The drawing under review shows one solid part. Ordinate dimensions are in mm from its lowest x, y, z. A direction names the side the tool comes from. Give positions to 0.01 mm unless a question says otherwise; leave off trailing zeros. Write each loop counter-clockwise with the first axis right and the second up, starting at its lowest first coordinate (ties: lowest second). Pieces come first, ordered by that corner, then holes. Notation, with made-up numbers: (-39.5, 16) -> (-31.5, 16) arc R35 ccw to (-31.5, 53) -> close; hole circle Ø4 at (-17.75, 17). An arc over 180 degrees is marked (long way). Answer as a JSON object with one key per item and string values.
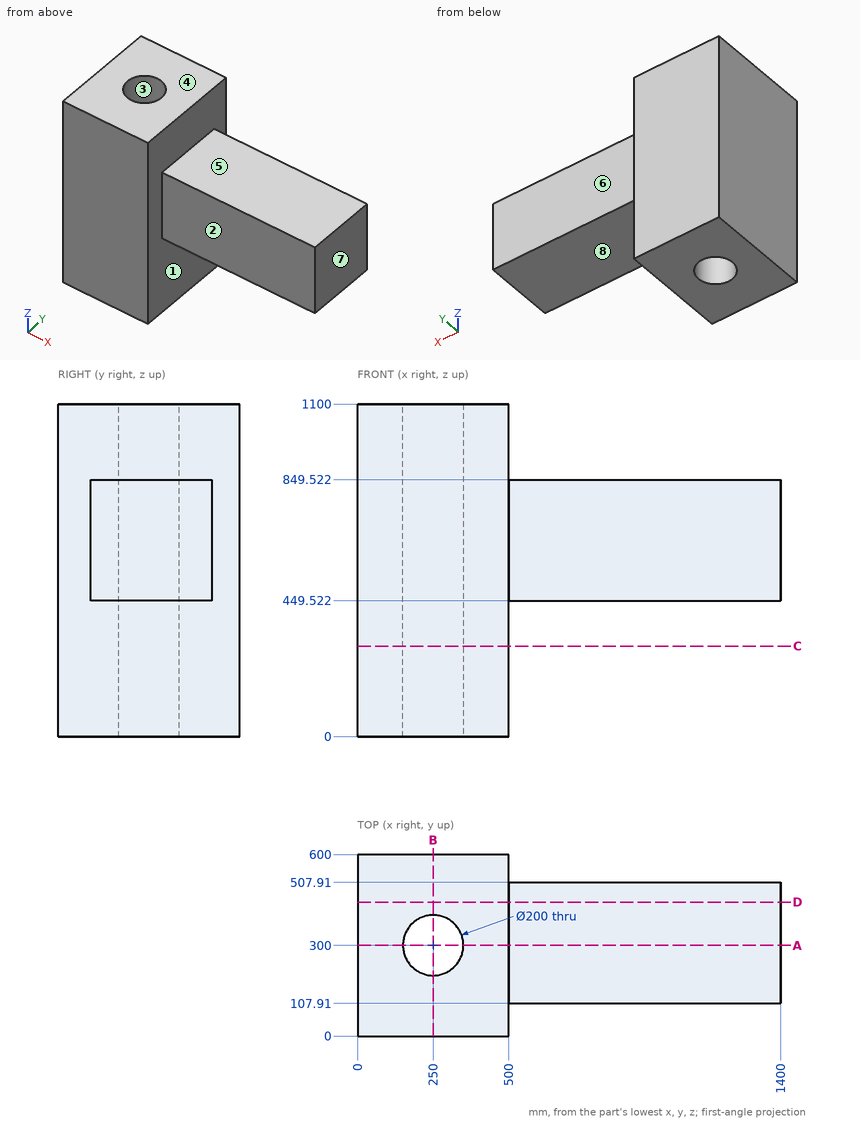
(1) For the marked faces 4, 5, 6, 7 and 8, list the 3-axis set-ups (+Z, -Z, +X, -X, +Y, -Y) from which the entire face can be reached by the end or side of a thin tool; tool diameter is ignored.
Here are the results:
{"face 4": "+Z, +X, -X, +Y, -Y", "face 5": "+Z, +X, +Y, -Y", "face 6": "+Z, -Z, +X, +Y", "face 7": "+Z, -Z, +X, +Y, -Y", "face 8": "-Z, +X, +Y, -Y"}
(2) For line 1 along Y through (x, z) = (250, 843); line 2 along X through (y, z) = (302.5, 296); line 3 along Z through (x, y) = (937, 423.5), list the stretches that pass through material, from the lowest coordinate up.
Here are the results:
{"line 1": "y = 0 to 200, 400 to 600", "line 2": "x = 0 to 150.03, 349.97 to 500", "line 3": "z = 449.52 to 849.52"}
(3) We need section D-D, the plane y = 443. State the section outline as (x, z) points.
Here are the results:
{"outline": "(0, 0) -> (500, 0) -> (500, 449.52) -> (1400, 449.52) -> (1400, 849.52) -> (500, 849.52) -> (500, 1100) -> (0, 1100) -> close"}
(4) The part is to be moulded in two halves that separate along Y. For the marked faces 1, 2 and 3, say which applies: +Y half, -Y half, draft (parallel to the pull), parting line (faces both ways), or undercut.
Here are the results:
{"face 1": "draft", "face 2": "-Y half", "face 3": "undercut"}
(5) We need section A-A, the plane y = 300. State the section outline as (x, z) points.
Here are the results:
{"outline": "(0, 0) -> (150, 0) -> (150, 1100) -> (0, 1100) -> close; (350, 0) -> (500, 0) -> (500, 449.52) -> (1400, 449.52) -> (1400, 849.52) -> (500, 849.52) -> (500, 1100) -> (350, 1100) -> close"}
(6) We need section C-C, the plane z = 299.5. State the section outline as (x, y) points.
Here are the results:
{"outline": "(0, 0) -> (500, 0) -> (500, 600) -> (0, 600) -> close; hole circle Ø200 at (250, 300)"}
(7) Clearance check with flat-ended pins moving along their axes: pin 1 (6 mm diameter, centred on x = 846, z = 743.5, fed in from +Y); pin 2 (6 mm diameter, centred on x = 696.5, y = 209.5, fed in from -Z); pin 3 (4 mm diameter, centred on x = 668, y = 431, fed in from +Z). State where each tip first meets the part, or that it passes through.
Here are the results:
{"pin 1": "stops at y = 507.91", "pin 2": "stops at z = 449.52", "pin 3": "stops at z = 849.52"}
(8) We need section B-B, the plane x = 250. State the section outline as (y, z) points, then the cut area to 3 significant figures.
Here are the results:
{"outline": "(0, 0) -> (200, 0) -> (200, 1100) -> (0, 1100) -> close; (400, 0) -> (600, 0) -> (600, 1100) -> (400, 1100) -> close", "area": "440,000 mm²"}
